```python
from build123d import *

# Parameters (mm, degrees)
F0_R     = 2.2479
F1_DEPTH = 27.94
F2_R     = 1.8288
F3_DEPTH = 33.3258
F4_DEPTH = 33.3258


with BuildPart() as f1:
    # F0 (on Front) → F1 (new body)
    with BuildSketch(Plane.XZ):
        Polygon((-36.4744, 18.648794), (-36.4744, -14.676006), (-34.8996, -14.676006), (-34.8996, 10.723994), (-28.5496, 10.723994), (-28.5496, -14.676006), (-26.9748, -14.676006), (-26.9748, 10.723994), (-20.6248, 10.723994), (-20.6248, -14.676006), (-19.05, -14.676006), (-19.05, 10.723994), (-12.7, 10.723994), (-12.7, -14.676006), (-11.1252, -14.676006), (-11.1252, 10.723994), (-4.7752, 10.723994), (-4.7752, -14.676006), (-3.2004, -14.676006), (-3.2004, 10.723994), (3.1496, 10.723994), (3.1496, -14.676006), (4.7244, -14.676006), (4.7244, 10.723994), (11.0744, 10.723994), (11.0744, -14.676006), (12.6492, -14.676006), (12.6492, 10.723994), (18.9992, 10.723994), (18.9992, -14.676006), (20.574, -14.676006), (20.574, 10.723994), (26.924, 10.723994), (26.924, -14.676006), (28.4988, -14.676006), (28.4988, 10.723994), (34.8488, 10.723994), (34.8488, -14.676006), (36.4744, -14.676006), (36.4744, 18.648794), align=None)
        with Locations((-23.8252, 14.127594)):
            Circle(F0_R, mode=Mode.SUBTRACT)
        with Locations((23.8252, 14.127594)):
            Circle(F0_R, mode=Mode.SUBTRACT)
    extrude(amount=F1_DEPTH)

    # F2 (on face) → F3 (cut, through all)
    with BuildSketch(Plane.XY.offset(18.648794)):
        with Locations((-31.115, -14.63412)):
            Circle(F2_R)
    extrude(amount=-F3_DEPTH, mode=Mode.SUBTRACT)

    # F2 (on face) → F4 (cut, through all)
    with BuildSketch(Plane.XY.offset(18.648794)):
        with Locations((31.115, -14.036736)):
            Circle(F2_R)
        with Locations((-31.115, -14.63412)):
            Circle(F2_R)
    extrude(amount=-F4_DEPTH, mode=Mode.SUBTRACT)


solid = f1.part
```
The listing builds one solid part. Answer for the finished solid, in the listing's coordinates (mm). A direction names the side the tool comes from. Give positions to 0.01 mm unless a question says otherwise; leave off trailing zeros. Write each loop counter-clockwise with the first axis right and the second up, starting at its lowest first coordinate (ties: lowest second). Pieces come first, ordered by that corner, then holes. Notation, with made-up numbers: (35.5, 55.25) -> (51.5, 55.25) arc R9 cw to (51.5, 61.25) -> close; hole circle Ø8 at (67.25, -9). An arc over 180 degrees is marked (long way). Write item = value, one per line. Start each with the question number.
1) The part is cut by section A-A, the plane z = 15.5. Determine the outline of the cut face in (x, y) (3 decimals), and give its area (3 significant figures).
2) Determine the mould class of faces 3 (the face through (-28, -14, -14.676)), 4 (the face through (3.15, -14, -2)) for opening direction X: +X half, -X half, draft (parallel to the pull), parting line (faces both ways), or undercut.
3) Straight lines are drawn through the part: line 1 along Z through (x, y) = (-24, -19.5); line 2 along X through (y, z) = (-7.75, 13.5); line 3 along Z through (x, y) = (-7, -15). For each, find the intervals that lie inside material, in ascending order.
4) Each of these flat-tipped pins is pushed along its axis until it touches: pin 1 (5 mm diameter, centred on x = -30.5, y = -13.5, fed in from -Z); pin 2 (1.5 mm diameter, centred on x = -14, z = -3, fed in from -Y); pin 3 (3 mm diameter, centred on x = 16.5, y = -9.5, fed in from -Z). Where does it stop, or does it pass through?
5) Which of the six approach directions +Z, -Z, +X, -X, +Y, -Y give full straight-line access (tool end or side, diameter ignored) to faces 1 (the face through (8, -14, 10.724)), 2 (the face through (-26.07, -13.77, 14.23))?
6) The part is cut by section C-C, the plane x = -15. Determine the outline of the cut face in (y, z).
7) The part is cut by section B-B, the plane z = 9. Count the separate pieces of the cut face and the enclosed holes in it, and give its area (3 significant figures).
Solutions:
q1.outline = (-36.474, -27.94) -> (-25.606, -27.94) -> (-25.606, 0) -> (-36.474, 0) -> close; (-22.045, -27.94) -> (22.045, -27.94) -> (22.045, 0) -> (-22.045, 0) -> close; (25.606, -27.94) -> (36.474, -27.94) -> (36.474, 0) -> (25.606, 0) -> close; hole circle Ø3.658 at (-31.115, -14.634); hole circle Ø3.658 at (31.115, -14.037)
q1.area = 1,820 mm²
q2.face_3 = draft
q2.face_4 = undercut
q3.line_1 = 10.72 to 11.89, 16.37 to 18.65
q3.line_2 = -36.47 to -25.98, -21.67 to 21.67, 25.98 to 36.47
q3.line_3 = 10.72 to 18.65
q4.pin_1 = -14.68
q4.pin_2 = through
q4.pin_3 = 10.72
q5.face_1 = -Z, +Y, -Y
q5.face_2 = +Y, -Y
q6.outline = (-27.94, 10.72) -> (0, 10.72) -> (0, 18.65) -> (-27.94, 18.65) -> close
q7.separate_pieces = 10
q7.enclosed_holes = 0
q7.area = 441 mm²
